Geometry: see drawing. Coordinates: mm, zero at the bounding-box minimum. A direction names the side the tool comes from. Give positions to 0.01 mm unless a question says otherwise; leave off trailing zeros. Write each loop counter-clockwise with the first axis right and the second up, starting at its lowest first coordinate (ties: lowest second). Pieces come first, ordered by that corner, then holes. Notation, with made-up numbers: (58, -18.75) - (77, -18.75) arc R17 ccw to (77, 1.25) - close; hole circle Ø8 at (65, 61). An arc over 180 degrees is marked (long way). Use CSV: the item, a comma, the result in double quotes. Start each with the question number.
(1) Section C-C on y = 17.5. Output: boundary loops of the cut face in (x, z) (1 decimal).
(2) First-contact query: pin 1 Ø10 at (x, z) = (38.5, 30) entering from +Y; pin 2 Ø5 at (y, z) = (8, 33.5) entering from +X (1 decimal); pin 3 Ø12 at (x, z) = (10.5, 119.5) entering from -Y. Flat tips, straight axial feed; report the tip coordinate or a pass-through.
(3) Section A-A on z = 156. Output: boundary loops of the cut face in (x, y).
(4) Reachability of the marked faces 1 and 2 from +Z, -Z, +X, -X, +Y, -Y: full face, straight path, thin tool, end or side. Return the list, or none.
(5) Section B-B on x = 12.5. Output: boundary loops of the cut face in (y, z), and give its area (3 significant figures).
(6) Line query: probe 1 along Y at (x, z) = (15, 130); probe 2 along Y at (x, z) = (15.5, 44) (1 decimal); probe 3 along X at (y, z) = (20.5, 162) (1 decimal). Output: solid intervals per line, ascending. Write a range as [from, to].
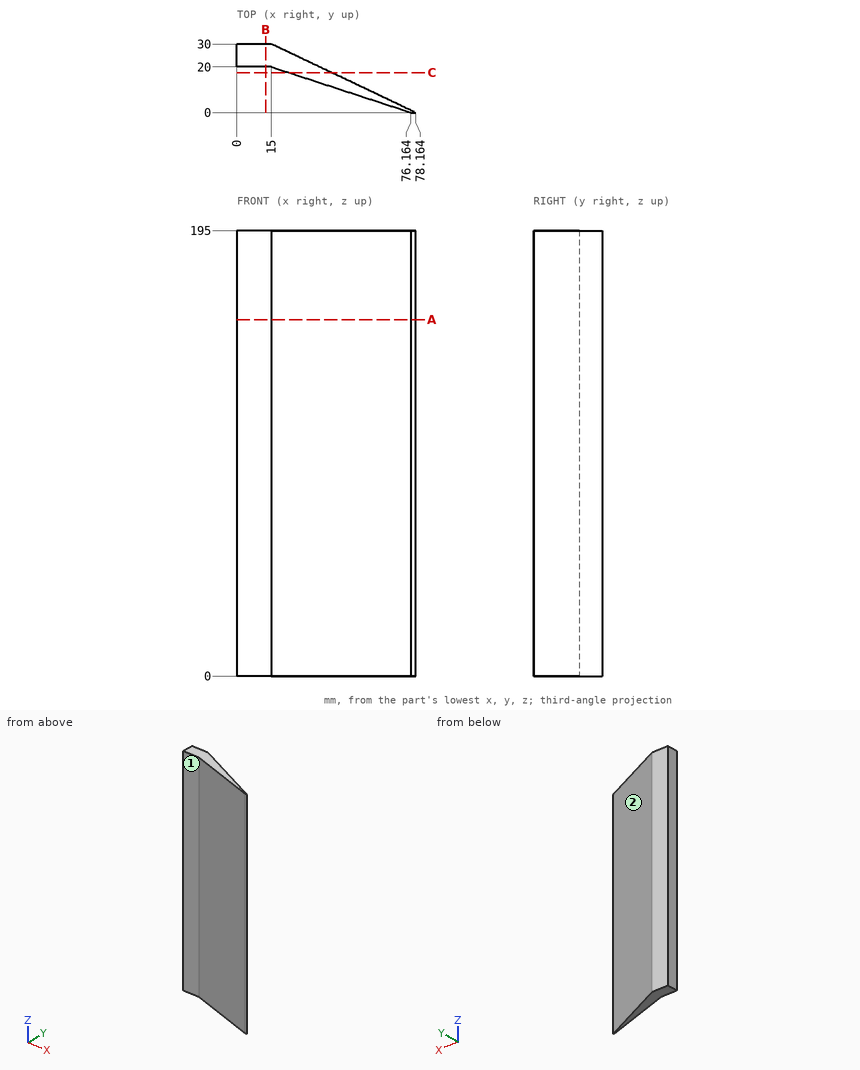
Check values:
1,outline,"(22.6, 0) - (41.3, 0) - (41.3, 195) - (22.6, 195) - close"
2,pin 1,"stops at y = 21.21"
2,pin 2,"stops at x = 66.6"
2,pin 3,"stops at y = 19.51"
3,outline,"(0, 20) - (15, 20) - (76.16, 0) - (78.16, 0) - (15, 30) - (0, 30) - close"
4,face 1,"+Z, -Z, -X, -Y"
4,face 2,"+Z, -Z, +X, +Y"
5,outline,"(20, 0) - (30, 0) - (30, 195) - (20, 195) - close"
5,area,"1,950 mm²"
6,probe 1,"y = [20, 30]"
6,probe 2,"y = [19.8, 29.8]"
6,probe 3,"x = [0, 35]"
